```python
from build123d import *

# Parameters (mm, degrees)
BOX005_W                    = 5
BOX005_H                    = 13
BOX005_DEPTH                = 4
BOX004_W                    = 3
BOX004_H                    = 31
BOX004_DEPTH                = 14
BOX003_W                    = 2
BOX003_H                    = 33
BOX003_DEPTH                = 11.2
BOX002_W                    = 3
BOX002_H                    = 35
BOX002_DEPTH                = 26
EXTRUDE_DEPTH               = 5
EXTRUDE001_DEPTH            = 5
THICKNESS_T                 = 1
BOX_W                       = 12
BOX_H                       = 31
BOX_DEPTH                   = 15
BOX001_W                    = 13
BOX001_H                    = 34
BOX001_DEPTH                = 14
CYLINDER001_W               = 48
CYLINDER001_H               = 15
CYLINDER001_ANGLE           = 60
CYLINDER001_PLACEMENT_ANGLE = 60
CYLINDER_W                  = 51
CYLINDER_H                  = 15
CYLINDER_ANGLE              = 60
CYLINDER_PLACEMENT_ANGLE    = 60


with BuildPart() as servo_wall_cutaway:
    # Box005 → Box005 (new body)
    with BuildSketch(Plane(origin=(-2, 19.5, 10), x_dir=(1, 0, 0), z_dir=(0, 0, 1))):
        with Locations((2.5, 6.5)):
            Rectangle(BOX005_W, BOX005_H)
    extrude(amount=BOX005_DEPTH)


with BuildPart() as slot_wall_cutout2:
    # Box004 → Box004 (new body)
    with BuildSketch(Plane(origin=(-1, 7, 14), x_dir=(1, 0, 0), z_dir=(0, 0, 1))):
        with Locations((1.5, 15.5)):
            Rectangle(BOX004_W, BOX004_H)
    extrude(amount=BOX004_DEPTH)


with BuildPart() as slot_wall_cutout1:
    # Box003 → Box003 (new body)
    with BuildSketch(Plane(origin=(-0.5, 6, 15), x_dir=(1, 0, 0), z_dir=(0, 0, 1))):
        with Locations((1, 16.5)):
            Rectangle(BOX003_W, BOX003_H)
    extrude(amount=BOX003_DEPTH)


with BuildPart() as wall_slot_finished:
    # Box002 → Box002 (new body)
    with BuildSketch(Plane(origin=(-1, 5, 0), x_dir=(1, 0, 0), z_dir=(0, 0, 1))):
        with Locations((1.5, 17.5)):
            Rectangle(BOX002_W, BOX002_H)
    extrude(amount=BOX002_DEPTH)

    # Cut003: cut slot wall cutout1
    add(slot_wall_cutout1.part, mode=Mode.SUBTRACT)

    # Cut004: cut slot wall cutout2
    add(slot_wall_cutout2.part, mode=Mode.SUBTRACT)


with BuildPart() as extrude_body:
    with BuildSketch(Plane(origin=(8.5, 45, 6), x_dir=(1, 0, 0), z_dir=(0, 1, 0))):
        with BuildLine():
            Line((5, 4), (-5, 4))
            Line((-5, 4), (-5, -3.142136))
            ThreePointArc((-5, -3.142136), (-2.53653, -3.783978), (0, -4))
            ThreePointArc((0, -4), (2.53653, -3.783978), (5, -3.142136))
            Line((5, -3.142136), (5, 4))
        make_face()
    extrude(amount=EXTRUDE_DEPTH)


with BuildPart() as extrude001:
    with BuildSketch(Plane(origin=(8.5, 45, 6), x_dir=(1, 0, 0), z_dir=(0, 1, 0))):
        with BuildLine():
            Line((5, 4), (-5, 4))
            Line((-5, 4), (-5, -3.142136))
            ThreePointArc((-5, -3.142136), (-2.53653, -3.783978), (0, -4))
            ThreePointArc((0, -4), (2.53653, -3.783978), (5, -3.142136))
            Line((5, -3.142136), (5, 4))
        make_face()
    extrude(amount=EXTRUDE001_DEPTH)


with BuildPart() as bolt_bottle_side_opening:
    # Thickness base: copy of Extrude body
    add(extrude_body.part)

    # Thickness
    thickness_openings = [bolt_bottle_side_opening.faces().sort_by_distance(p)[0] for p in [
        (8.5, 50, 5.862901),
    ]]
    offset(amount=THICKNESS_T, openings=thickness_openings)

    # Fusion: union Extrude body, Extrude001
    add(extrude_body.part)
    add(extrude001.part)


with BuildPart() as bolt_bottle_side_opening_1:
    # Fusion placement: moved
    add(bolt_bottle_side_opening.part.moved(Location((0, -7, 1))))


with BuildPart() as pullbay:
    # Box → Box (new body)
    with BuildSketch(Plane(origin=(2.5, 7, 2), x_dir=(1, 0, 0), z_dir=(0, 0, 1))):
        with Locations((6, 15.5)):
            Rectangle(BOX_W, BOX_H)
    extrude(amount=BOX_DEPTH)


with BuildPart() as cut_bay_from_case:
    # Box001 → Box001 (new body)
    with BuildSketch(Plane(origin=(2, 6, 0), x_dir=(1, 0, 0), z_dir=(0, 0, 1))):
        with Locations((6.5, 17)):
            Rectangle(BOX001_W, BOX001_H)
    extrude(amount=BOX001_DEPTH)

    # Cut001: cut pullBay
    add(pullbay.part, mode=Mode.SUBTRACT)


with BuildPart() as bottle_wall001:
    # Cylinder001 → Cylinder001 (revolve)
    with BuildSketch(Plane.XZ):
        with Locations((24, 7.5)):
            Rectangle(CYLINDER001_W, CYLINDER001_H)
    revolve(axis=Axis((0, 0, 0), (0, 0, 1)), revolution_arc=CYLINDER001_ANGLE)


with BuildPart() as bottle_wall001_1:
    # Cylinder001 placement: moved
    add(bottle_wall001.part.moved(Location((8.5, -7, 0))).rotate(Axis((8.5, -7, 0), (0, 0, 1)), CYLINDER001_PLACEMENT_ANGLE))


with BuildPart() as cut005:
    # Cylinder → Cylinder (revolve)
    with BuildSketch(Plane.XZ):
        with Locations((25.5, 7.5)):
            Rectangle(CYLINDER_W, CYLINDER_H)
    revolve(axis=Axis((0, 0, 0), (0, 0, 1)), revolution_arc=CYLINDER_ANGLE)


with BuildPart() as cut005_1:
    # Cylinder placement: moved
    add(cut005.part.moved(Location((8.5, -7, 0))).rotate(Axis((8.5, -7, 0), (0, 0, 1)), CYLINDER_PLACEMENT_ANGLE))

    # Cut: cut bottle_wall001
    add(bottle_wall001_1.part, mode=Mode.SUBTRACT)


with BuildPart() as cut005_2:
    # Cut placement: moved
    add(cut005_1.part.moved(Location((0, -2, 0))))

    # Fusion001: union cut bay from case
    add(cut_bay_from_case.part)

    # Cut002: cut bolt_bottle_side_opening
    add(bolt_bottle_side_opening_1.part, mode=Mode.SUBTRACT)

    # Fusion002: union wall slot finished
    add(wall_slot_finished.part)

    # Cut005: cut servo wall cutaway
    add(servo_wall_cutaway.part, mode=Mode.SUBTRACT)


solid = cut005_2.part
```
Here's how the part is built. I have some questions about the finished solid (model axes, mm). A direction names the side the tool comes from. Round coordinates to 2 decimals unless told otherwise and drop trailing zeros. Loops run counter-clockwise (first coordinate to the right, second up) from the corner with the lowest first, then second, coordinate; pieces in that order, holes last.
1. Suppose I cut it at A-A, the plane z = 17. Please give me the cut outline in (x, y), and give its area (3 significant figures).
Answers:
outline: (-1, 5) - (2, 5) - (2, 7) - (1.5, 7) - (1.5, 6) - (-0.5, 6) - (-0.5, 7) - (-1, 7) - close; (-1, 38) - (-0.5, 38) - (-0.5, 39) - (1.5, 39) - (1.5, 38) - (2, 38) - (2, 40) - (-1, 40) - close
area: 8.00 mm2
2. Will these pins go through, and if not, where does the flat tip stop? pin 1 (3.5 mm diameter, centred on x = 0.5, z = 19, fed in from +Y); pin 2 (0.5 mm diameter, centred on x = 14, z = 2.5, fed in from -Y); pin 3 (0.8 mm diameter, centred on y = 38.5, z = 19, fed in from -X); pin 4 (1.5 mm diameter, centred on x = 17, y = 28.5, fed in from +Z).
Answers:
pin 1: stops at y = 40
pin 2: stops at y = 6
pin 3: stops at x = -1
pin 4: passes through
3. Suppose I cut it at B-B, the plane y = 28. Please give me the cut outline in (x, z).
Answers:
outline: (-1, 0) - (15, 0) - (15, 14) - (14.5, 14) - (14.5, 2) - (2.5, 2) - (2.5, 10) - (-1, 10) - close
4. For faces 1 (the face through (1, 19.5, 12)), 2 (the face through (0.5, 39.2, 26)), 3 (the face through (15, 22, 7)), 4 (the face through (0, 6, 20)), 5 (the face through (8, 28, 0)), which set-ups out of +Z, -Z, +X, -X, +Y, -Y let a thin tool reach every point of the face, with its end or its side?
Answers:
face 1: +Z, -X
face 2: +Z, +X, -X, +Y, -Y
face 3: +Z, -Z, -Y
face 4: +Z
face 5: -Z, +X, -X, +Y, -Y
5. Suppose I cut it at D-D, the plane y = 37. Please give me the cut outline in (x, z).
Answers:
outline: (-13.52, 0) - (-5.21, 0) - (-5.21, 15) - (-13.52, 15) - close; (-1, 0) - (15, 0) - (15, 14) - (14.5, 14) - (14.5, 2) - (2.5, 2) - (2.5, 14) - (-1, 14) - close; (22.21, 0) - (30.52, 0) - (30.52, 15) - (22.21, 15) - close
6. Thinking about a two-plate mould opening in Y: for faces 6 (the face through (2, 6, 16)), 7 (the face through (0, 5, 13)), 8 (the face through (1, 32.5, 12)), 9 (the face through (0, 40, 20)), which applies, released by +Y, released by -Y, zero draft, split by the parting line, or undercut?
Answers:
face 6: zero draft
face 7: released by -Y
face 8: undercut
face 9: released by +Y
7. Suppose I cut it at C-C, the plane z = 5. Please give me the cut outline in (x, y), and give its area (3 significant figures).
Answers:
outline: (-17, 35.17) - (-15.5, 32.57) arc R48 cw to (-1, 38.05) - (-1, 5) - (2, 5) - (2, 6) - (15, 6) - (15, 38.56) arc R48 cw to (32.5, 32.57) - (34, 35.17) arc R51 ccw to (14.5, 41.65) - (14.5, 7) - (2.5, 7) - (2.5, 41.65) arc R51 ccw to start
area: 264 mm2
8. If I drill on probe 1 along X at (y, z) = (32.5, 4); probe 2 along X at (y, z) = (33, 13); probe 3 along X at (y, z) = (33.5, 5.5), over which ranges is the centre line in solid material (lowest first)?
Answers:
probe 1: x = -1 to 2.5, 14.5 to 15
probe 2: x = -15.75 to -14.74, -1 to 2.5, 14.5 to 15, 31.74 to 32.75
probe 3: x = -16.04 to -13.81, -1 to 2.5, 14.5 to 15, 30.81 to 33.04
